For this review, use the dimensioned drawing (mm, ordinates from the lowest corner) and the shaded views. A direction names the side the tool comes from. Give positions to 0.01 mm unless a question says otherwise; leave off trailing zeros. Loops run counter-clockwise (first coordinate to the right, second up) from the corner with the lowest first, then second, coordinate; pieces in that order, holes last. Notation, with made-up numbers: (-28, 52) - (-2, 52) arc R17 cw to (-2, 62) - close; hole circle Ø2 at (2, -24.75). An arc over 180 degrees is marked (long way). Put each result on its own line as item: value.
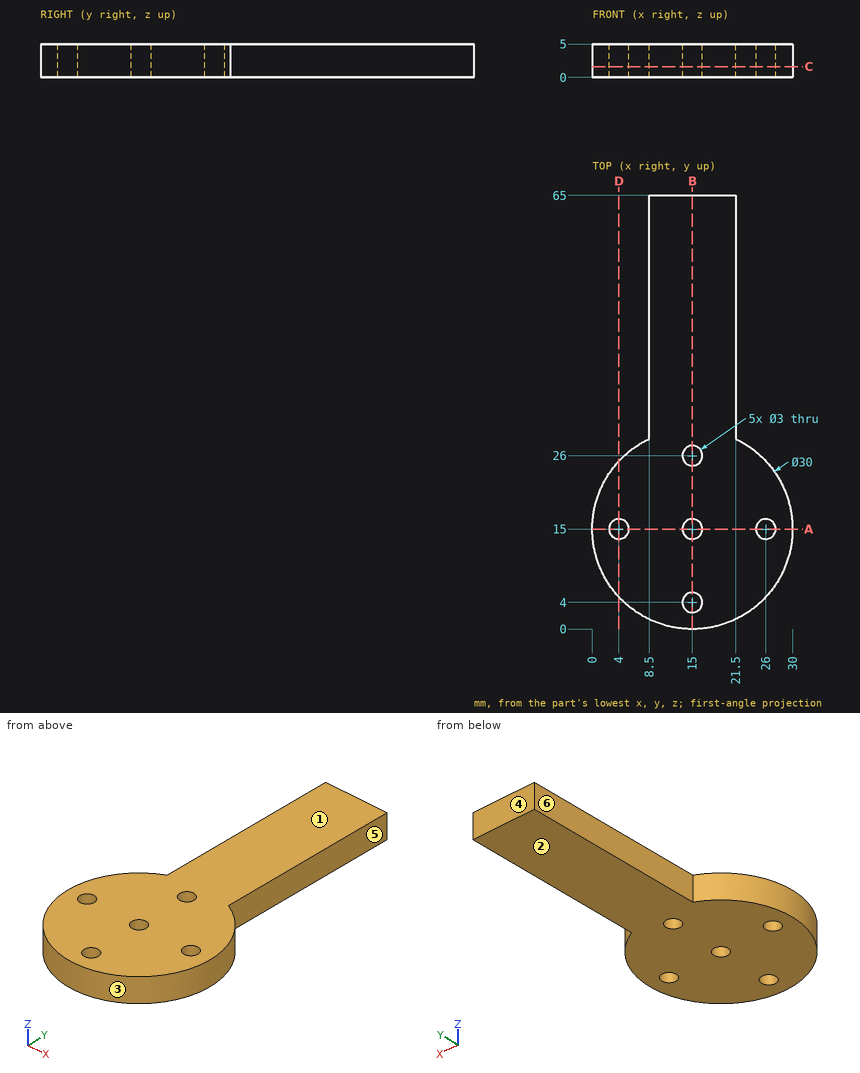
1) Insertion check: pin 1 Ø2.5 at (x, y) = (26, 15) entering from +Z; pin 2 Ø1.5 at (x, z) = (18.5, 4.5) entering from -Y; pin 3 Ø3 at (x, z) = (10, 2) entering from -Y; pin 4 Ø5 at (x, y) = (15, 26) entering from +Z. Each pin has a flat end and moves straight along its axis. Give the tip position at first contact, or say it passes through.
Geometry check:
pin 1: passes through
pin 2: stops at y = 0.25
pin 3: stops at y = 0.41
pin 4: stops at z = 5
2) Draft analysis for pull direction Z (two halves, no side actions). For the marked faces 1, 2 and 3, state which applies: pulls with the +Z half, pulls with the -Z half, needs draft (parallel to the pull), parting line crosses it, or undercut.
Geometry check:
face 1: pulls with the +Z half
face 2: pulls with the -Z half
face 3: needs draft
3) Take a section at B-B on x = 15. State the section outline as (y, z) points, and give its area (3 significant figures).
Geometry check:
outline: (0, 0) - (2.5, 0) - (2.5, 5) - (0, 5) - close; (5.5, 0) - (13.5, 0) - (13.5, 5) - (5.5, 5) - close; (16.5, 0) - (24.5, 0) - (24.5, 5) - (16.5, 5) - close; (27.5, 0) - (65, 0) - (65, 5) - (27.5, 5) - close
area: 280 mm²
4) Take a section at C-C on z = 1.6. State the section outline as (x, y) points.
Geometry check:
outline: (8.5, 28.52) arc R15 ccw (long way) to (21.5, 28.52) - (21.5, 65) - (8.5, 65) - close; hole circle Ø3 at (4, 15); hole circle Ø3 at (15, 4); hole circle Ø3 at (15, 15); hole circle Ø3 at (15, 26); hole circle Ø3 at (26, 15)
5) Wall thickness on line 1 (Y direction, x = 15, z = 3.7); line 2 (Y direction, x = 15.75, z = 4); line 3 (X direction, y = 40, z = 1.65): over which ranges is each line inside the solid? List them lowest first.
Geometry check:
line 1: y = 0 to 2.5, 5.5 to 13.5, 16.5 to 24.5, 27.5 to 65
line 2: y = 0.02 to 2.7, 5.3 to 13.7, 16.3 to 24.7, 27.3 to 65
line 3: x = 8.5 to 21.5
6) For the marked faces 4, 5 and 6, list the 3-axis set-ups (+Z, -Z, +X, -X, +Y, -Y) from which the entire face can be reached by the end or side of a thin tool; tool diameter is ignored.
Geometry check:
face 4: +Z, -Z, +X, -X, +Y
face 5: +Z, -Z, +X, +Y
face 6: +Z, -Z, -X, +Y
7) Take a section at D-D on x = 4. State the section outline as (y, z) points.
Geometry check:
outline: (4.8, 0) - (13.5, 0) - (13.5, 5) - (4.8, 5) - close; (16.5, 0) - (25.2, 0) - (25.2, 5) - (16.5, 5) - close
8) Take a section at A-A on y = 15. State the section outline as (x, z) points.
Geometry check:
outline: (0, 0) - (2.5, 0) - (2.5, 5) - (0, 5) - close; (5.5, 0) - (13.5, 0) - (13.5, 5) - (5.5, 5) - close; (16.5, 0) - (24.5, 0) - (24.5, 5) - (16.5, 5) - close; (27.5, 0) - (30, 0) - (30, 5) - (27.5, 5) - close
